Part model, mm, in its own coordinate system. Coordinates: 2 decimals unless noted, no trailing zeros. Loops run counter-clockwise (first coordinate to the right, second up) from the corner with the lowest first, then second, coordinate; pieces in that order, holes last. Notation, with made-up numbers: (35, 81.25) -> (39, 81.25) arc R30 ccw to (39, 112.25) -> close; hole circle Ø11 at (27.25, 42.5). An arc over 180 degrees is marked (long way). One line per question, with ' | ' between items. Start each with the question number.
1) Cut at D-D (x = 135). List the corners of the cut face in (y, z), plus the area to 3 significant figures.
2) Probe L1, parallel to X at y = 2.95, z = 0; L2, parallel to Z at x = 24, y = 2.9; L3, parallel to X at y = 2.4, z = 223. List the from-to ranges inside material, lowest first. Write a range as from..to.
3) Cut at A-A (z = 0). List the corners of the cut face in (x, y).
4) Two-plate mould, pull along Z, no slides. Class faces 1 (the face through (225.56, 1.97, -107.81)), 2 (the face through (-39.05, 2.03, -8.67)), 3 (the face through (224.922, 1.972, 109.134)): released by +Z, released by -Z, zero draft, split by the parting line, or undercut.
5) Cut at C-C (z = 70). List the corners of the cut face in (x, y).
6) Drop flat-ended pins along their axis: pin 1 (0.9 mm diameter, centred on x = 0, y = 1, fed in from -Z); pin 2 (1 mm diameter, centred on x = 17.5, y = 1, fed in from -Z); pin 3 (2 mm diameter, centred on y = 3, z = 10.5, fed in from -X). Give the stop position or say it passes through.
7) Cut at B-B (y = 1.85). Count the separate pieces of the cut face and the enclosed holes in it, plus the area to 3 significant figures.
from build123d import *

# Parameters (mm, degrees)
SKETCH1_R                = 250
BOSS_EXTRUDE1_DEPTH      = 4
CUT_EXTRUDE5_DEPTH       = 4
FILLET1_R                = 1
CIRPATTERN1_COUNT        = 14
FILLET1_OF_CIRPATTERN1_R = 1
SKETCH12_R               = 40
CUT_EXTRUDE6_DEPTH       = 10
SKETCH16_W               = 100
SKETCH16_H               = 4
CUT_EXTRUDE10_DEPTH      = 100


with BuildPart() as part:
    # Sketch1 → Boss-Extrude1 (new body)
    with BuildSketch(Plane(origin=(0, 0, 0), x_dir=(1, 0, 0), z_dir=(0, 1, 0))):
        with Locations(Location((0, 0, 0), (0, 0, 270))):
            Circle(SKETCH1_R)
    extrude(amount=BOSS_EXTRUDE1_DEPTH)

    # Sketch11 → Cut-Extrude5 (cut)
    with BuildSketch(Plane(origin=(0, 4, 0), x_dir=(1, 0, 0), z_dir=(0, 1, 0))):
        with BuildLine():
            Line((1.5, 245), (-1.5, 245))
            ThreePointArc((-1.5, 245), (-2.207106781, 245.292893219), (-2.5, 246))
            Line((-2.5, 246), (-2.5, 255))
            Line((-2.5, 255), (2.5, 255))
            Line((2.5, 255), (2.5, 246))
            ThreePointArc((2.5, 246), (2.207106781, 245.292893219), (1.5, 245))
        make_face()
    cut_extrude5 = extrude(amount=-CUT_EXTRUDE5_DEPTH, mode=Mode.SUBTRACT)

    # Fillet1
    fillet1_edges = [part.edges().sort_by_distance(p)[0] for p in [
        (-2.5, 2, -249.987499687),
        (2.5, 2, -249.987499687),
    ]]
    fillet(fillet1_edges, radius=FILLET1_R)

    # CirPattern1: Cut-Extrude5 ×14 about axis
    cirpattern1_axis = Axis((0, 0, 0), (0, 1, 0))
    for i in range(1, CIRPATTERN1_COUNT):
        add(cut_extrude5.rotate(cirpattern1_axis, i * 360 / CIRPATTERN1_COUNT), mode=Mode.SUBTRACT)

    # Fillet1 of CirPattern1
    fillet1_of_cirpattern1_edges = [part.edges().sort_by_distance(p)[0] for p in [
        (-110.717933267, 2, -224.146245235),
        (-106.213088927, 2, -226.315663931),
        (-197.006821984, 2, -153.910077941),
        (-193.889372974, 2, -157.819235353),
        (-244.276093477, 2, -53.190132127),
        (-243.163488807, 2, -58.064771688),
        (-243.163488807, 2, 58.064771688),
        (-244.276093477, 2, 53.190132127),
        (-193.889372974, 2, 157.819235353),
        (-197.006821984, 2, 153.910077941),
        (-106.213088927, 2, 226.315663931),
        (-110.717933267, 2, 224.146245235),
        (2.5, 2, 249.987499687),
        (-2.5, 2, 249.987499687),
        (110.717933267, 2, 224.146245235),
        (106.213088927, 2, 226.315663931),
        (197.006821984, 2, 153.910077941),
        (193.889372974, 2, 157.819235353),
        (244.276093477, 2, 53.190132127),
        (243.163488807, 2, 58.064771688),
        (243.163488807, 2, -58.064771688),
        (244.276093477, 2, -53.190132127),
        (193.889372974, 2, -157.819235353),
        (197.006821984, 2, -153.910077941),
        (106.213088927, 2, -226.315663931),
        (110.717933267, 2, -224.146245235),
    ]]
    fillet(fillet1_of_cirpattern1_edges, radius=FILLET1_OF_CIRPATTERN1_R)

    # Sketch12 → Cut-Extrude6 (cut)
    with BuildSketch(Plane(origin=(0, 4, 0), x_dir=(1, 0, 0), z_dir=(0, 1, 0))):
        with Locations(Location((0, 0, 0), (0, 0, 270))):
            Circle(SKETCH12_R)
    extrude(amount=-CUT_EXTRUDE6_DEPTH, mode=Mode.SUBTRACT)

    # Sketch16 → Cut-Extrude10 (cut)
    with BuildSketch(Plane(origin=(0, 4, 0), x_dir=(1, 0, 0), z_dir=(0, 1, 0))):
        with Locations((0, 200)):
            Rectangle(SKETCH16_W, SKETCH16_H)
    extrude(amount=-CUT_EXTRUDE10_DEPTH, mode=Mode.SUBTRACT)


solid = part.part
Reported:
1) outline: (0, -210.42) -> (4, -210.42) -> (4, 210.42) -> (0, 210.42) -> close | area: 1,680 mm²
2) L1: x = -250..-40, 40..250 | L2: z = -248.85..-202, -198..-32, 32..248.85 | L3: x = -113.01..-110.17, -104.62..104.62, 110.17..113.01
3) outline: (-250, 0) -> (-40, 0) -> (-40, 4) -> (-250, 4) -> close; (40, 0) -> (250, 0) -> (250, 4) -> (40, 4) -> close
4) face 1: released by -Z | face 2: undercut | face 3: released by +Z
5) outline: (-240, 0) -> (240, 0) -> (240, 4) -> (-240, 4) -> close
6) pin 1: stops at z = -245 | pin 2: stops at z = -249.42 | pin 3: stops at x = -249.82
7) separate pieces: 1 | enclosed holes: 2 | area: 191,000 mm²
